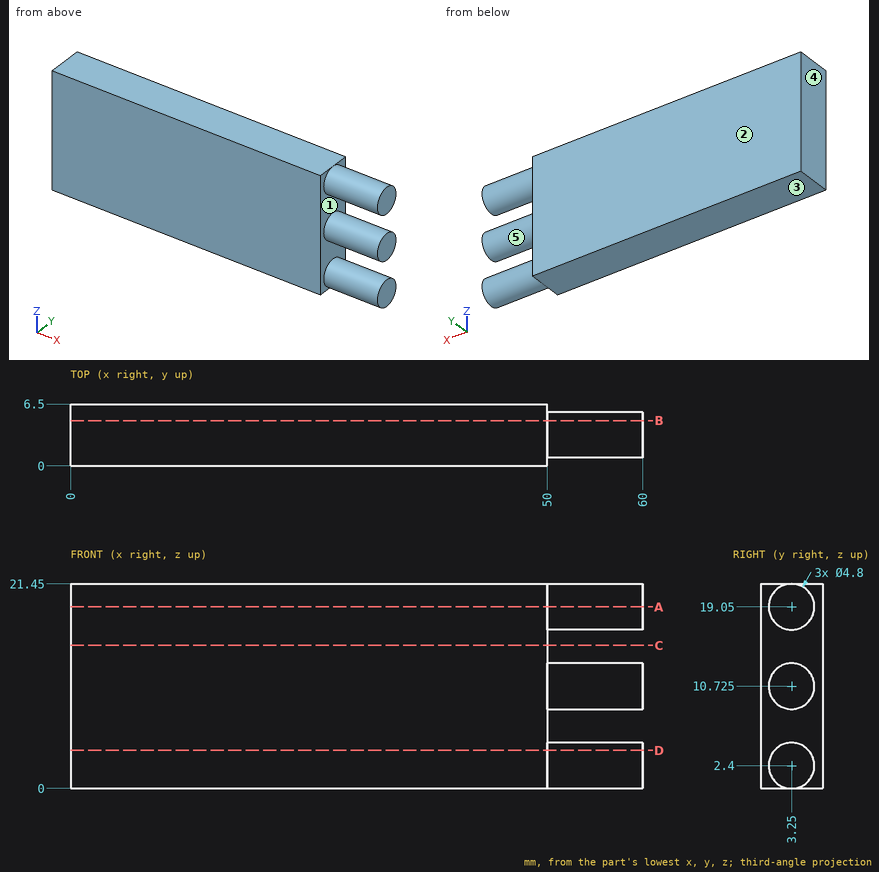
The drawing under review shows one solid part. Ordinate dimensions are in mm from its lowest x, y, z. A direction names the side the tool comes from. Give positions to 0.01 mm unless a question says otherwise; leave off trailing zeros. Order: outer loops, then holes, each group sorted by start corner. A loop starts at its lowest first (then second) coordinate and runs counter-clockwise, first axis right, second up. Notation, with made-up numbers: (-18, 79) -> (29, 79) arc R19 cw to (29, 90) -> close; hole circle Ø10 at (-25, 10.5). An arc over 180 degrees is marked (long way). Write item = value, one per line. Start each with the question number.
(1) To check wall thickness, follow line 1 along Z through (x, y) = (50.5, 3.75); line 2 along X through (y, z) = (1.25, 9). State the ranges of each line that lie inside material, in increasing order.
(2) We need section A-A on z = 19.05. Write out the cut boundary in (x, y).
(3) We need section C-C on z = 15. Write out the cut boundary in (x, y), plus the area to 3 significant figures.
(4) Mouldability with a two-part tool opening along Z and no side actions: class the marked faces 3, 4 and 5 as +Z half, -Z half, draft (parallel to the pull), parting line (faces both ways), or undercut.
(5) We need section B-B on y = 4.75. Write out the cut boundary in (x, z), plus the area to 3 significant figures.
(6) We need section D-D on z = 4. Write out the cut boundary in (x, y), plus the area to 3 significant figures.
(7) For the marked faces 1 and 2, list the 3-axis set-ups (+Z, -Z, +X, -X, +Y, -Y) from which the entire face can be reached by the end or side of a thin tool; tool diameter is ignored.
Numbers:
q1.line_1 = 0.05 to 4.75, 8.38 to 13.07, 16.7 to 21.4
q1.line_2 = 0 to 50
q2.outline = (0, 0) -> (50, 0) -> (50, 0.85) -> (60, 0.85) -> (60, 5.65) -> (50, 5.65) -> (50, 6.5) -> (0, 6.5) -> close
q3.outline = (0, 0) -> (50, 0) -> (50, 6.5) -> (0, 6.5) -> close
q3.area = 325 mm^2
q4.face_3 = -Z half
q4.face_4 = draft
q4.face_5 = undercut
q5.outline = (0, 0) -> (50, 0) -> (50, 0.53) -> (60, 0.53) -> (60, 4.27) -> (50, 4.27) -> (50, 8.85) -> (60, 8.85) -> (60, 12.6) -> (50, 12.6) -> (50, 17.18) -> (60, 17.18) -> (60, 20.92) -> (50, 20.92) -> (50, 21.45) -> (0, 21.45) -> close
q5.area = 1,180 mm^2
q6.outline = (0, 0) -> (50, 0) -> (50, 1.46) -> (60, 1.46) -> (60, 5.04) -> (50, 5.04) -> (50, 6.5) -> (0, 6.5) -> close
q6.area = 361 mm^2
q7.face_1 = +X
q7.face_2 = +Z, -Z, +X, -X, +Y
